Geometry check sheet. Reference: the model listing, model coordinates, mm. Face numbers are marked on the shaded views. A direction names the side the tool comes from. Give positions to 0.01 mm unless a question says otherwise; leave off trailing zeros. Write each loop counter-clockwise with the first axis right and the second up, starting at its lowest first coordinate (ties: lowest second). Pieces come first, ordered by that corner, then holes. Notation, with made-up numbers: M 56.5,15 L 94.5,15 A17 ccw 94.5,48 Z; hole C -32.5,-29 d6. An arc over 180 degrees is marked long. One line per item, written item: value. Start each with the question number.
1. Cross-section at C-C on y = 25.5. Record the cut outline in (x, z).
2. Cross-section at A-A on z = 0. Record the cut outline in (x, y).
3. Cross-section at B-B on x = -33. Record the cut outline in (y, z).
4. Scan lines: line 1 (Z direction, x = -108, y = 4); line 2 (Y direction, x = -40, z = 0.75); line 3 (X direction, y = 53, z = -2). Record each from-to range of solid material in increasing order.
5. Gauge pin test, flat ends, axial feed: pin 1 (10 mm diameter, centred on x = -58, z = -3, fed in from +Y); pin 2 (12 mm diameter, centred on y = 68.5, z = -0.5, fed in from -X). Record the tip position at first contact, or that the pin passes through.
6. Tool access check on the marked faces 1 and 2. Record the directions out of +Z, -Z, +X, -X, +Y, -Y that give a thin tool (end or side, any length) a straight path to the whole face; none if there is none.
from build123d import *

# Parameters (mm, degrees)
PAD_DEPTH    = 10
SKETCH001_R  = 2.6
POCKET_DEPTH = 175.001


with BuildPart() as part:
    # Sketch → Pad (new body, symmetric)
    with BuildSketch(Plane.XY):
        with BuildLine():
            Line((0, 175), (-8, 175))
            Line((-8, 175), (-8, 23))
            ThreePointArc((-23, 8), (-12.393398, 12.393398), (-8, 23))
            Line((-23, 8), (-125, 8))
            Line((-125, 8), (-125, 0))
            Line((-125, 0), (-23, 0))
            ThreePointArc((-23, 0), (-6.736544, 6.736544), (0, 23))
            Line((0, 23), (0, 175))
        make_face()
    extrude(amount=PAD_DEPTH, both=True)

    # Sketch001 → Pocket (cut, through all)
    with BuildSketch(Plane.XZ):
        with Locations((-108, 0)):
            Circle(SKETCH001_R)
        with Locations((-33, 0)):
            Circle(SKETCH001_R)
    extrude(amount=-POCKET_DEPTH, mode=Mode.SUBTRACT)


solid = part.part
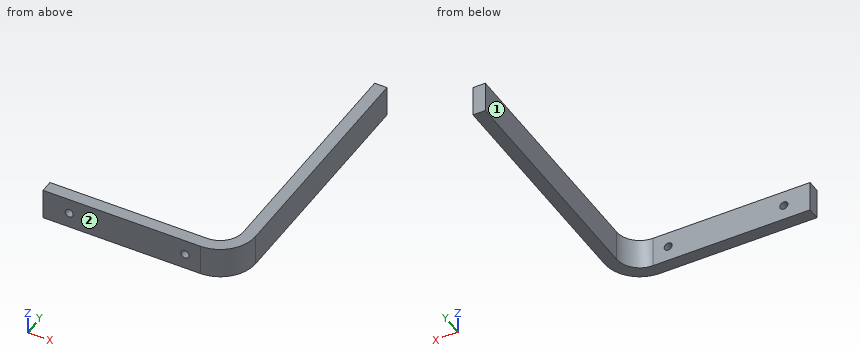
Report:
1. outline: M -8,-10 L 0,-10 L 0,10 L -8,10 Z
2. outline: M -125,0 L -110.6,0 L -110.6,8 L -125,8 Z; M -105.4,0 L -35.6,0 L -35.6,8 L -105.4,8 Z; M -30.4,0 L -23,0 A23 ccw 0,23 L 0,175 L -8,175 L -8,23 A15 cw -23,8 L -30.4,8 Z
3. outline: M 0,-10 L 8,-10 L 8,-2.6 L 0,-2.6 Z; M 0,2.6 L 8,2.6 L 8,10 L 0,10 Z
4. line 1: z = -10 to -2.6, 2.6 to 10
4. line 2: y = 0 to 8
4. line 3: x = -8 to 0
5. pin 1: stops at y = 8
5. pin 2: stops at x = -8
6. face 1: +Z, -Z, -X, +Y
6. face 2: +Z, -Z, +X, -X, -Y
